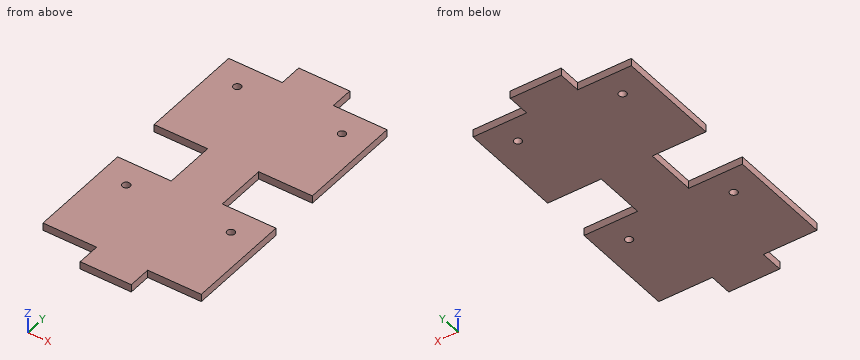
```python
from build123d import *

# Parameters (mm, degrees)
CROQUIS2_W              = 21
CROQUIS2_H              = 41
CROQUIS2_R              = 1.5
SALIENTE_EXTRUIR1_DEPTH = 3


with BuildPart() as part:
    # Croquis2 → Saliente-Extruir1 (new body)
    # profile 1 of 5: a face of its own
    with BuildSketch(Plane.XY):
        with Locations((20.5, 33.908588505)):
            Rectangle(CROQUIS2_W, CROQUIS2_H)
        with Locations((20.5, 44.408588505)):
            Circle(CROQUIS2_R, mode=Mode.SUBTRACT)
    # profile 2 of 5: a face of its own
    with BuildSketch(Plane.XY):
        Polygon((-10, 63.408588505), (-10, -56.591411495), (0, -56.591411495), (10, -56.591411495), (10, 63.408588505), align=None)
    # profile 3 of 5: a face of its own
    with BuildSketch(Plane.XY):
        with Locations((-20.5, 33.908588505)):
            Rectangle(CROQUIS2_W, CROQUIS2_H)
        with Locations((-20.5, 44.408588505)):
            Circle(CROQUIS2_R, mode=Mode.SUBTRACT)
    # profile 4 of 5: a face of its own
    with BuildSketch(Plane.XY):
        with Locations((-20.5, -27.091411495)):
            Rectangle(CROQUIS2_W, CROQUIS2_H)
        with Locations((-20.5, -16.591411495)):
            Circle(CROQUIS2_R, mode=Mode.SUBTRACT)
    # profile 5 of 5: a face of its own
    with BuildSketch(Plane.XY):
        with Locations((20.5, -27.091411495)):
            Rectangle(CROQUIS2_W, CROQUIS2_H)
        with Locations((20.5, -16.591411495)):
            Circle(CROQUIS2_R, mode=Mode.SUBTRACT)
    extrude(amount=SALIENTE_EXTRUIR1_DEPTH)


solid = part.part
```
The listing builds one solid part. Answer for the finished solid, in the listing's coordinates (mm). Coordinates: 2 decimals unless noted, no trailing zeros. Write each loop counter-clockwise with the first axis right and the second up, starting at its lowest first coordinate (ties: lowest second). Pieces come first, ordered by that corner, then holes. Notation, with made-up numbers: M 46,81 L 58,81 A6 cw 58,87 Z; hole C 32,19 d1. An arc over 180 degrees is marked long. Use a Markdown table: item, result. Add a question column.
1. Section A-A (x = 13) is taken. Give the vertices of the cut face in (y, z).
2. Section B-B (x = 20.5) is taken. Give the vertices of the cut face in (y, z).
3. Straight lines are drawn through the part: line 1 along Y through (x, z) = (-20.5, 2.25); line 2 along Y through (x, z) = (-24, 0.8); line 3 along X through (y, z) = (45, 2.9). For each, find the intervals that lie inside material, in ascending order. Write a range as [from, to].
4. Section C-C (z = 0.75) is taken. Give the vertices of the cut face in (x, y).
5. Given P1, Ø0.9, axis at y = 60.5, z = 2, coming from the -X side; P2, Ø1.5, axis at y = 0, z = 2, coming from the +X side; P3, Ø0.9, axis at x = -20.5, z = 1.5, coming from the -Y side, each flat-ended and moving along its own axis, determine where each tip first touches the part or whether it passes through.
Data:
| question | item | result |
|---|---|---|
| 1 | outline | M -47.59,0 L -6.59,0 L -6.59,3 L -47.59,3 Z; M 13.41,0 L 54.41,0 L 54.41,3 L 13.41,3 Z |
| 2 | outline | M -47.59,0 L -18.09,0 L -18.09,3 L -47.59,3 Z; M -15.09,0 L -6.59,0 L -6.59,3 L -15.09,3 Z; M 13.41,0 L 42.91,0 L 42.91,3 L 13.41,3 Z; M 45.91,0 L 54.41,0 L 54.41,3 L 45.91,3 Z |
| 3 | line 1 | y = [-47.59, -18.09], [-15.09, -6.59], [13.41, 42.91], [45.91, 54.41] |
| 3 | line 2 | y = [-47.59, -6.59], [13.41, 54.41] |
| 3 | line 3 | x = [-31, -21.88], [-19.12, 19.12], [21.88, 31] |
| 4 | outline | M -31,-47.59 L -10,-47.59 L -10,-56.59 L 10,-56.59 L 10,-47.59 L 31,-47.59 L 31,-6.59 L 10,-6.59 L 10,13.41 L 31,13.41 L 31,54.41 L 10,54.41 L 10,63.41 L -10,63.41 L -10,54.41 L -31,54.41 L -31,13.41 L -10,13.41 L -10,-6.59 L -31,-6.59 Z; hole C -20.5,-16.59 d3; hole C -20.5,44.41 d3; hole C 20.5,-16.59 d3; hole C 20.5,44.41 d3 |
| 5 | P1 | stops at x = -10 |
| 5 | P2 | stops at x = 10 |
| 5 | P3 | stops at y = -47.59 |
